from build123d import *

# Parameters (mm, degrees)
SKETCH_1_W            = 100
SKETCH_1_H            = 300
EXTRUDE_1_DEPTH       = 4
EXTRUDE_2_DEPTH       = 442
SKETCH_3_W            = 50
SKETCH_3_H            = 300
EXTRUDE_3_DEPTH       = 4
HOLE_WIZARD_4_0_4_1_D = 4


with BuildPart() as part:
    # 草图1 → 凸台-拉伸1 (new body)
    with BuildSketch(Plane(origin=(0, 0, 0), x_dir=(1, 0, 0), z_dir=(0, 1, 0))):
        with Locations((50, 150)):
            Rectangle(SKETCH_1_W, SKETCH_1_H)
    extrude(amount=EXTRUDE_1_DEPTH)

    # 草图2 → 凸台-拉伸2 (add)
    with BuildSketch(Plane(origin=(0, 4, 0), x_dir=(1, 0, 0), z_dir=(0, 1, 0))):
        Polygon((0, 0), (8.236039078, 0), (50, 0), (50, 3.5), (4, 3.5), (4, 296.5), (50, 296.5), (50, 300), (8.236039078, 300), (0, 300), align=None)
    extrude(amount=EXTRUDE_2_DEPTH)

    # 草图3 → 凸台-拉伸3 (add)
    with BuildSketch(Plane(origin=(0, 446, 0), x_dir=(1, 0, 0), z_dir=(0, 1, 0))):
        with Locations((25, 150)):
            Rectangle(SKETCH_3_W, SKETCH_3_H)
    extrude(amount=EXTRUDE_3_DEPTH)

    # Ø4.0 (4) 直径孔1 (through all)
    with Locations(Plane(origin=(0, 0, 0), x_dir=(-1, 0, 0), z_dir=(0, -1, 0))):
        with Locations((-60, 13.5), (-60, 286.5)):
            Hole(HOLE_WIZARD_4_0_4_1_D / 2)


solid = part.part
Check sheet for the modelled part. Datum: model origin and axes. Units: mm. A direction names the side the tool comes from. Give positions to 0.01 mm unless a question says otherwise; leave off trailing zeros. Order: outer loops, then holes, each group sorted by start corner. A loop starts at its lowest first (then second) coordinate and runs counter-clockwise, first axis right, second up. Notation, with made-up numbers: M 45,11 L 79,11 A13 ccw 79,28 Z; hole C 67,-21.5 d5. An arc over 180 degrees is marked long. Answer as CSV lines item,"result". Start each with the question number.
Item 1: Thickness scan on line 1 (Y direction, x = 6.5, z = -115.5); line 2 (Z direction, x = 60, y = 1.4); line 3 (Z direction, x = 24, y = 168). Record the ranges inside material, lowest first. Write a range as [from, to].
Item 2: Gauge pin test, flat ends, axial feed: P1, Ø1.5, axis at y = 147, z = -233.5, coming from the +X side; P2, Ø4.5, axis at x = 60, z = -286.5, coming from the +Y side. Record the tip position at first contact, or that the pin passes through.
Item 3: Cross-section at C-C on x = 90. Enter the section's corners in (y, z), plus the area to 3 significant figures.
Item 4: Cross-section at B-B on y = 311.5. Enter the section's corners in (x, z), plus the area to 3 significant figures.
Item 5: Cross-section at A-A on z = -122.5. Enter the section's corners in (x, y).
Item 6: Tool access check on faces 1 (the face through (27, 222, 0)), 2 (the face through (4, 222, -148)). Record the directions out of +Z, -Z, +X, -X, +Y, -Y that give a thin tool (end or side, any length) a straight path to the whole face; none if there is none.
Item 7: Mould release check, pull along Z, two halves, no side actions. Record for faces 3 (the face through (25, 450, -152)), 4 (the face through (27, 222, -296.5)), 5 (the face through (27, 222, -300)), 6 (the face through (27, 222, -3.5)): +Z half, -Z half, draft (parallel to the pull), parting line (faces both ways), or undercut.
Established:
1,line 1,"y = [0, 4], [446, 450]"
1,line 2,"z = [-300, -288.5], [-284.5, -15.5], [-11.5, 0]"
1,line 3,"z = [-300, -296.5], [-3.5, 0]"
2,P1,"stops at x = 4"
2,P2,"stops at y = 4"
3,outline,"M 0,-300 L 4,-300 L 4,0 L 0,0 Z"
3,area,"1,200 mm^2"
4,outline,"M 0,-300 L 50,-300 L 50,-296.5 L 4,-296.5 L 4,-3.5 L 50,-3.5 L 50,0 L 0,0 Z"
4,area,"1,520 mm^2"
5,outline,"M 0,0 L 100,0 L 100,4 L 4,4 L 4,446 L 50,446 L 50,450 L 0,450 Z"
6,face 1,"+Z, +X, -X, +Y, -Y"
6,face 2,"+X"
7,face 3,"draft"
7,face 4,"undercut"
7,face 5,"-Z half"
7,face 6,"undercut"
